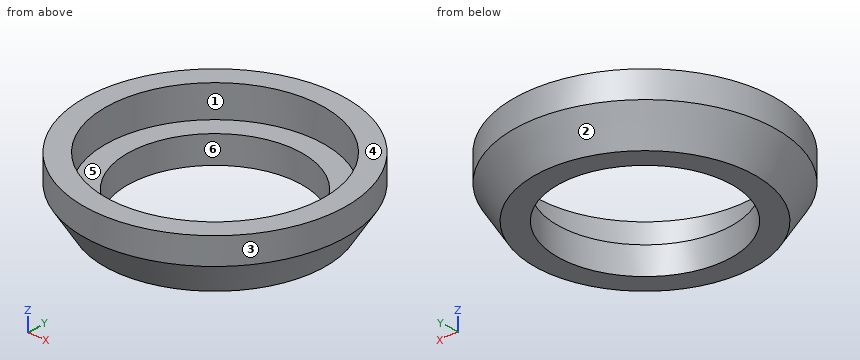
from build123d import *

# Parameters (mm, degrees)
SKETCH1_R             = 9.525
BOSS_EXTRUDE1_DEPTH   = 4.5
SKETCH2_R             = 6.35
CUT_EXTRUDE1_DEPTH    = 10
CHAMFER1_SIZE         = 1.5
CHAMFER1_SIZE2        = 2.400501794
CHAMFER1_PART_2_SIZE  = 1.5
CHAMFER1_PART_2_SIZE2 = 2.400501794
SKETCH3_R             = 7.874
CUT_EXTRUDE2_DEPTH    = 2.011
SKETCH4_R             = 7.94385
CUT_EXTRUDE3_DEPTH    = 4.98
SKETCH5_R             = 24.237402282
CUT_EXTRUDE4_DEPTH    = 5.5
SKETCH6_R             = 11.614236141
CUT_EXTRUDE5_DEPTH    = 0.15


with BuildPart() as part:
    # Sketch1 → Boss-Extrude1 (new body, symmetric)
    with BuildSketch(Plane.XY):
        Circle(SKETCH1_R)
    extrude(amount=BOSS_EXTRUDE1_DEPTH, both=True)

    # Sketch2 → Cut-Extrude1 (cut, through all)
    with BuildSketch(Plane.XY.offset(4.5)):
        Circle(SKETCH2_R)
    extrude(amount=-CUT_EXTRUDE1_DEPTH, mode=Mode.SUBTRACT)

    # Chamfer1
    chamfer1_edges = [part.edges().sort_by_distance(p)[0] for p in [
        (-9.525, 0, -4.5),
    ]]
    chamfer1_side = [part.faces().sort_by_distance(p)[0] for p in [
        (-9.255592316, 0, -4.5),
    ]]
    chamfer(chamfer1_edges, length=CHAMFER1_SIZE, length2=CHAMFER1_SIZE2, reference=chamfer1_side[0])

    # Chamfer1 part 2
    chamfer1_part_2_edges = [part.edges().sort_by_distance(p)[0] for p in [
        (-9.525, 0, 4.5),
    ]]
    chamfer1_part_2_side = [part.faces().sort_by_distance(p)[0] for p in [
        (-9.255592316, 0, 4.5),
    ]]
    chamfer(chamfer1_part_2_edges, length=CHAMFER1_PART_2_SIZE, length2=CHAMFER1_PART_2_SIZE2, reference=chamfer1_part_2_side[0])

    # Sketch3 → Cut-Extrude2 (cut)
    with BuildSketch(Plane.XY.offset(4.5)):
        Circle(SKETCH3_R)
    extrude(amount=-CUT_EXTRUDE2_DEPTH, mode=Mode.SUBTRACT)

    # Sketch4 → Cut-Extrude3 (cut)
    with BuildSketch(Plane.XY.offset(2.489)):
        Circle(SKETCH4_R)
    extrude(amount=-CUT_EXTRUDE3_DEPTH, mode=Mode.SUBTRACT)

    # Sketch5 → Cut-Extrude4 (cut, through all)
    with BuildSketch(Plane.XY):
        Circle(SKETCH5_R)
    extrude(amount=CUT_EXTRUDE4_DEPTH, mode=Mode.SUBTRACT)

    # Sketch6 → Cut-Extrude5 (cut)
    with BuildSketch(Plane.XY):
        Circle(SKETCH6_R)
    extrude(amount=-CUT_EXTRUDE5_DEPTH, mode=Mode.SUBTRACT)


solid = part.part
Source: CAD feature listing. Evaluate the final solid. Frame: model axes, mm. Face numbers are marked on the shaded views. A direction names the side the tool comes from. Give positions to 0.01 mm unless a question says otherwise; leave off trailing zeros. Order: outer loops, then holes, each group sorted by start corner. A loop starts at its lowest first (then second) coordinate and runs counter-clockwise, first axis right, second up. Notation, with made-up numbers: (24, -23) -> (64, -23) arc R21 cw to (64, 0) -> close; hole circle Ø1 at (0, -34). An arc over 180 degrees is marked (long way). Write item = value, one per line.
Q1. Cut plane C-C, the plane z = -1.4. Output: boundary loops of the cut face in (x, y) (3 decimals).
Data:
outline = circle Ø19.05 at (0, 0); hole circle Ø15.888 at (0, 0)
Q2. Pin query (flat end, axial travel): pin 1 (2 mm diameter, centred on y = -2, z = -3.5, fed in from -X); pin 2 (8 mm diameter, centred on x = 3, y = -2, fed in from +Z); pin 3 (1 mm diameter, centred on x = 3.5, z = -3.5, fed in from +Y). Return the tip coordinate at first contact, or that it passes through.
Data:
pin_1 = -9.09
pin_2 = -2.49
pin_3 = 8.31
Q3. Material intervals for line 1 (Y direction, x = -0.25, z = -0.65); line 2 (Y direction, x = 6.25, z = -1); line 3 (X direction, y = -5, z = -3.5), sorted ascending. Write a range as from..to.
Data:
line_1 = -9.52..-7.94, 7.94..9.52
line_2 = -7.19..-4.9, 4.9..7.19
line_3 = -7.06..-3.91, 3.91..7.06
Q4. Cut plane D-D, the plane z = -3.6. Output: boundary loops of the cut face in (x, y).
Data:
outline = circle Ø17.17 at (0, 0); hole circle Ø12.7 at (0, 0)
Q5. Pull-direction query (Y, two-part tool) for the marked faces 3, 4, 5 and 6; classes: released by +Y, released by -Y, zero draft, split by the parting line, or undercut.
Data:
face_3 = split by the parting line
face_4 = zero draft
face_5 = undercut
face_6 = undercut
Q6. Set-up query: the marked faces 1 and 2. Return all of +Z, -Z, +X, -X, +Y, -Y with unobstructed straight access to the full face (end or side cutting, diameter ignored); none if empty.
Data:
face_1 = +Z
face_2 = -Z
